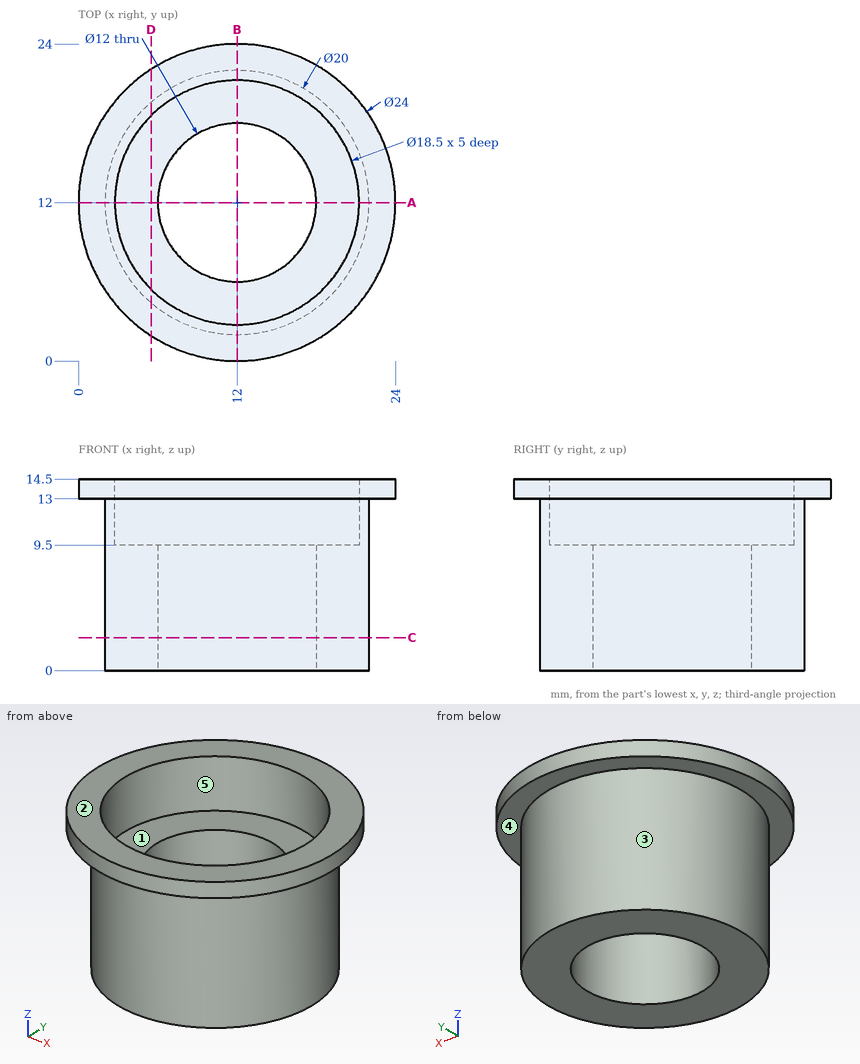
The figure shows three views and two pictorial views of one solid part (mm, origin at its lowest corner). Answer the questions. A direction names the side the tool comes from. Coordinates: 2 decimals unless noted, no trailing zeros. Loops run counter-clockwise (first coordinate to the right, second up) from the corner with the lowest first, then second, coordinate; pieces in that order, holes last.
1) Find section A-A on y = 12. Write down the section's boundary in (x, z), then the cut area to 3 significant figures.
2) Determine the mould class of the marked faces 3, 4 and 5 for opening direction X: pulls with the +X half, pulls with the -X half, needs draft (parallel to the pull), parting line crosses it, or undercut.
3) Find section C-C on z = 2.5. Write down the section's boundary in (x, y), then the cut area to 3 significant figures.
4) Find the intervals of material crossed by L1, parallel to Y at x = 12, z = 12.8; L2, parallel to Y at x = 12, z = 5.25; L3, parallel to Z at x = 10.25, y = 1, in increasing order.
5) Find section D-D on x = 5.5. Write down the section's boundary in (y, z), then the cut area to 3 significant figures.
6) Flat-ended cylindrical pins translate along their axes: pin 1 Ø6 at (x, z) = (10, 3.5) entering from -Y; pin 2 Ø3 at (y, z) = (6.5, 8.5) entering from -X; pin 3 Ø6 at (x, z) = (5, 5.5) entering from +Y. Find the tip coordinate at first contact, or state that the pin passes through.
7) A tool of negligible diameter and unlimited length cuts with its end or side. For the marked faces 1 and 2, from which of +Z, -Z, +X, -X, +Y, -Y can it reach the whole face along a straight path? Write none if from no direction.
Values:
1. outline: (0, 13) - (2, 13) - (2, 0) - (6, 0) - (6, 9.5) - (2.75, 9.5) - (2.75, 14.5) - (0, 14.5) - close; (18, 0) - (22, 0) - (22, 13) - (24, 13) - (24, 14.5) - (21.25, 14.5) - (21.25, 9.5) - (18, 9.5) - close
1. area: 89.5 mm2
2. face 3: parting line crosses it
2. face 4: needs draft
2. face 5: undercut
3. outline: circle Ø20 at (12, 12); hole circle Ø12 at (12, 12)
3. area: 201 mm2
4. L1: y = 2 to 2.75, 21.25 to 22
4. L2: y = 2 to 6, 18 to 22
4. L3: z = 13 to 14.5
5. outline: (1.91, 13) - (4.4, 13) - (4.4, 0) - (19.6, 0) - (19.6, 13) - (22.09, 13) - (22.09, 14.5) - (18.58, 14.5) - (18.58, 9.5) - (5.42, 9.5) - (5.42, 14.5) - (1.91, 14.5) - close
5. area: 162 mm2
6. pin 1: stops at y = 2
6. pin 2: stops at x = 2.83
6. pin 3: stops at y = 21.17
7. face 1: +Z
7. face 2: +Z, +X, -X, +Y, -Y
